```python
from build123d import *

# Parameters (mm, degrees)
SKETCH1_W           = 50
SKETCH1_H           = 100
BOSS_EXTRUDE1_DEPTH = 20
SKETCH2_W           = 4
SKETCH2_H           = 20
CUT_EXTRUDE1_DEPTH  = 20
SKETCH3_W           = 4
SKETCH3_H           = 20
CUT_EXTRUDE2_DEPTH  = 16
SKETCH4_W           = 5
SKETCH4_H           = 60
CUT_EXTRUDE3_DEPTH  = 114.578166916
SKETCH6_R           = 1.75
CUT_EXTRUDE5_DEPTH  = 114.578166916
SKETCH7_R           = 4
CUT_EXTRUDE6_DEPTH  = 5
SKETCH8_R           = 3.25
CUT_EXTRUDE7_DEPTH  = 2.5
SKETCH9_W           = 50
SKETCH9_H           = 20
BOSS_EXTRUDE2_DEPTH = 15
SKETCH5_R           = 1.75
CUT_EXTRUDE4_DEPTH  = 113.805141727


with BuildPart() as part:
    # Sketch1 → Boss-Extrude1 (new body)
    with BuildSketch(Plane.XY):
        with Locations((25, 50)):
            Rectangle(SKETCH1_W, SKETCH1_H)
    extrude(amount=BOSS_EXTRUDE1_DEPTH)

    # Sketch2 → Cut-Extrude1 (cut)
    with BuildSketch(Plane.ZY):
        with Locations((11, 80)):
            Rectangle(SKETCH2_W, SKETCH2_H)
    cut_extrude1 = extrude(amount=-CUT_EXTRUDE1_DEPTH, mode=Mode.SUBTRACT)

    # Sketch3 → Cut-Extrude2 (cut)
    with BuildSketch(Plane.XY.offset(20)):
        with Locations((18, 80)):
            Rectangle(SKETCH3_W, SKETCH3_H)
    cut_extrude2 = extrude(amount=-CUT_EXTRUDE2_DEPTH, mode=Mode.SUBTRACT)

    # Mirror1: Cut-Extrude1, Cut-Extrude2 across plane
    add(cut_extrude1.mirror(Plane.ZY.offset(-25)), mode=Mode.SUBTRACT)
    add(cut_extrude2.mirror(Plane.ZY.offset(-25)), mode=Mode.SUBTRACT)

    # Sketch4 → Cut-Extrude3 (cut, through all)
    with BuildSketch(Plane.ZY):
        with Locations((17.5, 30)):
            Rectangle(SKETCH4_W, SKETCH4_H)
    extrude(amount=-CUT_EXTRUDE3_DEPTH, mode=Mode.SUBTRACT)

    # Sketch6 → Cut-Extrude5 (cut, through all)
    with BuildSketch(Plane.XY.offset(20)):
        with BuildLine():
            ThreePointArc((19.25, 61), (16.975951413, 62.66969251), (16.063859338, 60))
            Line((16.063859338, 60), (18.936140662, 60))
            ThreePointArc((18.936140662, 60), (19.16969251, 60.475951413), (19.25, 61))
        make_face()
        with BuildLine():
            Line((18.936140662, 60), (16.063859338, 60))
            ThreePointArc((16.063859338, 60), (17.5, 59.25), (18.936140662, 60))
        make_face()
        with BuildLine():
            ThreePointArc((34.25, 61), (31.975951413, 62.66969251), (31.063859338, 60))
            Line((31.063859338, 60), (33.936140662, 60))
            ThreePointArc((33.936140662, 60), (34.16969251, 60.475951413), (34.25, 61))
        make_face()
        with BuildLine():
            Line((33.936140662, 60), (31.063859338, 60))
            ThreePointArc((31.063859338, 60), (32.5, 59.25), (33.936140662, 60))
        make_face()
        with Locations((32.5, 41)):
            Circle(SKETCH6_R)
        with Locations((17.5, 41)):
            Circle(SKETCH6_R)
    extrude(amount=-CUT_EXTRUDE5_DEPTH, mode=Mode.SUBTRACT)

    # Sketch7 → Cut-Extrude6 (cut)
    with BuildSketch(Plane.XY.offset(20)):
        with Locations((32.5, 61)):
            Circle(SKETCH7_R)
        with Locations((17.5, 61)):
            Circle(SKETCH7_R)
    extrude(amount=-CUT_EXTRUDE6_DEPTH, mode=Mode.SUBTRACT)

    # Sketch8 → Cut-Extrude7 (cut)
    with BuildSketch(Plane.XY.offset(15)):
        with Locations((17.5, 61)):
            Circle(SKETCH8_R)
        with Locations((32.5, 61)):
            Circle(SKETCH8_R)
        with Locations((32.5, 41)):
            Circle(SKETCH8_R)
        with Locations((17.5, 41)):
            Circle(SKETCH8_R)
    extrude(amount=-CUT_EXTRUDE7_DEPTH, mode=Mode.SUBTRACT)

    # Sketch9 → Boss-Extrude2 (add)
    with BuildSketch(Plane.XY.offset(15)):
        with Locations((25, -10)):
            Rectangle(SKETCH9_W, SKETCH9_H)
    extrude(amount=-BOSS_EXTRUDE2_DEPTH)

    # Sketch5 → Cut-Extrude4 (cut, through all)
    with BuildSketch(Plane.XY.offset(15)):
        with Locations((34.1, 15)):
            Circle(SKETCH5_R)
        with Locations((15.9, -5)):
            Circle(SKETCH5_R)
    extrude(amount=-CUT_EXTRUDE4_DEPTH, mode=Mode.SUBTRACT)


solid = part.part
```
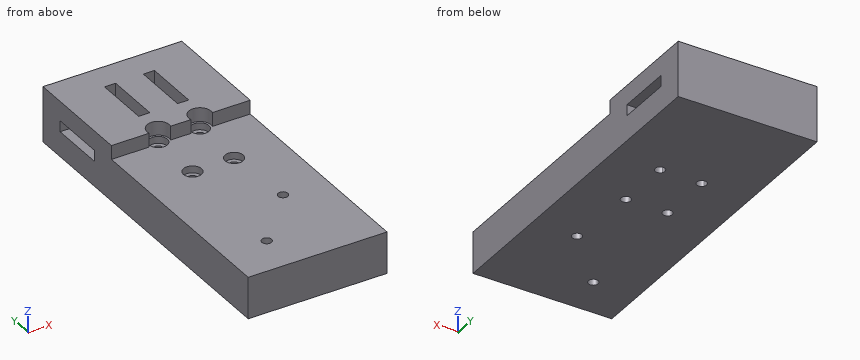
Model file for the job. Use its own axes, mm. Coordinates: 2 decimals unless noted, no trailing zeros. Loops run counter-clockwise (first coordinate to the right, second up) from the corner with the lowest first, then second, coordinate; pieces in that order, holes last. Notation, with made-up numbers: (-21.75, 77) - (19.25, 77) arc R11 ccw to (19.25, 93) - close; hole circle Ø5 at (-35, 4). An arc over 180 degrees is marked (long way). Answer as a JSON object with one key per item and string values. Group by question number.
(1) Cut at D-D (x = 5). Give the cut face in (y, z), then the cut area to 3 significant figures.
(2) Cut at A-A (y = 41). Give the cut face in (x, z), then the cut area to 3 significant figures.
(3) Cut at B-B (y = 15). Give the cut face in (x, z), then the cut area to 4 significant figures.
(4) Flat gauge pins, fed straight in: pin 1 (7 mm diameter, centred on x = 17, y = 40.5, fed in from +Z); pin 2 (4.5 mm diameter, centred on x = 32.5, y = 61, fed in from +Z); pin 3 (2.5 mm diameter, centred on x = 23.5, z = 18.5, fed in from -Y). Where does each tip first touch, or does it go through?
(5) Cut at C-C (z = 18.25). Give the cut face in (x, y), then the cut area to 3 significant figures.
(6) Probe line 1 along X through (y, z) = (61, 18.3); line 2 along Z through (x, y) = (15, 80); line 3 along X through (y, z) = (71.5, 6.25). List the from-to ranges inside material, lowest first.
Geometry says:
{
 "1": {"outline": "(-20, 0) - (100, 0) - (100, 20) - (60, 20) - (60, 15) - (-20, 15) - close; hole (70, 9) - (90, 9) - (90, 13) - (70, 13) - close", "area": "1,920 mm^2"},
 "2": {"outline": "(0, 0) - (15.75, 0) - (15.75, 12.5) - (14.25, 12.5) - (14.25, 15) - (0, 15) - close; (19.25, 0) - (30.75, 0) - (30.75, 12.5) - (29.25, 12.5) - (29.25, 15) - (20.75, 15) - (20.75, 12.5) - (19.25, 12.5) - close; (34.25, 0) - (50, 0) - (50, 15) - (35.75, 15) - (35.75, 12.5) - (34.25, 12.5) - close", "area": "630 mm^2"},
 "3": {"outline": "(0, 0) - (32.35, 0) - (32.35, 15) - (0, 15) - close; (35.85, 0) - (50, 0) - (50, 15) - (35.85, 15) - close", "area": "697.5 mm^2"},
 "4": {"pin 1": "stops at z = 15", "pin 2": "stops at z = 12.5", "pin 3": "stops at y = 60"},
 "5": {"outline": "(0, 60) - (13.63, 60) arc R4 cw (long way) to (21.37, 60) - (28.63, 60) arc R4 cw (long way) to (36.37, 60) - (50, 60) - (50, 100) - (0, 100) - close; hole (16, 70) - (20, 70) - (20, 90) - (16, 90) - close; hole (30, 70) - (34, 70) - (34, 90) - (30, 90) - close", "area": "1,770 mm^2"},
 "6": {"line 1": "x = 0 to 13.5, 21.5 to 28.5, 36.5 to 50", "line 2": "z = 0 to 9, 13 to 20", "line 3": "x = 0 to 16, 20 to 30, 34 to 50"}
}
